Can you work these out from the model? Positions are in its coordinate system, mm. A direction names the side the tool comes from. Give positions to 0.01 mm unless a question says otherwise; leave off trailing zeros. Loops run counter-clockwise (first coordinate to the right, second up) from the corner with the lowest first, then second, coordinate; pieces in that order, holes last. Notation, with made-up numbers: (-37.75, 4) - (-7.75, 4) arc R30 ccw to (-7.75, 42) - close; hole circle Ø6 at (68, 88). An arc over 180 degrees is marked (long way). Answer as a JSON object with one key per item and string values. Group by question number.
Item 1: Suppose I cut it at B-B on x = 45.5. Write out the boundary of the cut face in (y, z), and give its area (3 significant figures).
Item 2: Suppose I cut it at A-A on y = 7.25. Write out the boundary of the cut face in (x, z), and give its area (3 significant figures).
Item 3: Thinking about a two-plate mould opening in X: for faces 1 (the flat face through (94.975, 10, 0)), 2 (the flat face through (78, 10, 25)), 3 (the flat face through (61.975, 10, 0)), which applies, pulls with the +X half, pulls with the -X half, needs draft (parallel to the pull), parting line crosses it, or undercut?
Item 4: Suppose I cut it at D-D on x = 8. Write out the boundary of the cut face in (y, z).
Item 5: Which directions (+Z, -Z, +X, -X, +Y, -Y) give clear straight access to the entire face, cutting with the end or side of a thin tool? Please do faces 4 (the flat face through (26.475, 10, 0)), 5 (the flat face through (78, 10, -25)), 6 (the flat face through (42, 10, 23)).
Item 6: Will these pins go through, and if not, where does the flat tip stop? pin 1 (5 mm diameter, centred on y = 9, z = -6.5, fed in from -X); pin 2 (3 mm diameter, centred on x = 73.5, y = 9, fed in from -Z); pin 3 (3 mm diameter, centred on y = 9, z = 9.5, fed in from +X).
Item 7: Suppose I cut it at C-C on z = 11.5. Write out the boundary of the cut face in (x, y).
Item 8: Please list where these lines run through material, in increasing order: L1, parallel to X at y = 8.75, z = 2.5; L2, parallel to Z at x = -33.5, y = 11.25; L3, parallel to Z at x = 43.5, y = 11.
from build123d import *

# Parameters (mm, degrees)
SKETCH1_W           = 165
SKETCH1_H           = 65
BOSS_EXTRUDE1_DEPTH = 5
FILLET1_R           = 5
SKETCH2_W           = 82
SKETCH2_H           = 55
SKETCH2_W_2         = 31
SKETCH2_H_2         = 46
SKETCH2_W_3         = 33
SKETCH2_H_3         = 50
BOSS_EXTRUDE2_DEPTH = 10
FILLET2_R           = 2
FILLET3_R           = 1


with BuildPart() as part:
    # Sketch1 → Boss-Extrude1 (new body)
    with BuildSketch(Plane(origin=(0, 0, 0), x_dir=(1, 0, 0), z_dir=(0, 1, 0))):
        with Locations((17.474934091, 0)):
            Rectangle(SKETCH1_W, SKETCH1_H)
    extrude(amount=BOSS_EXTRUDE1_DEPTH)

    # Fillet1
    fillet1_edges = [part.edges().sort_by_distance(p)[0] for p in [
        (-65.025065909, 2.5, -32.5),
        (99.974934091, 2.5, -32.5),
        (99.974934091, 2.5, 32.5),
        (-65.025065909, 2.5, 32.5),
    ]]
    fillet(fillet1_edges, radius=FILLET1_R)

    # Sketch2 → Boss-Extrude2 (add)
    with BuildSketch(Plane(origin=(0, 5, 0), x_dir=(1, 0, 0), z_dir=(0, 1, 0))):
        with Locations((-19.025065909, 0)):
            Rectangle(SKETCH2_W, SKETCH2_H)
        with Locations((41.974934091, 0)):
            Rectangle(SKETCH2_W_2, SKETCH2_H_2)
        with Locations((78.474934091, 0)):
            Rectangle(SKETCH2_W_3, SKETCH2_H_3)
    extrude(amount=BOSS_EXTRUDE2_DEPTH)

    # Fillet2
    fillet2_edges = [part.edges().sort_by_distance(p)[0] for p in [
        (26.474934091, 10, -23),
        (26.474934091, 10, 23),
        (57.474934091, 10, 23),
        (57.474934091, 10, -23),
    ]]
    fillet(fillet2_edges, radius=FILLET2_R)

    # Fillet3
    fillet3_edges = [part.edges().sort_by_distance(p)[0] for p in [
        (61.974934091, 10, -25),
        (61.974934091, 10, 25),
        (94.974934091, 10, 25),
        (94.974934091, 10, -25),
    ]]
    fillet(fillet3_edges, radius=FILLET3_R)


solid = part.part
Worked out:
{
 "1": {"outline": "(0, -32.5) - (5, -32.5) - (5, -23) - (15, -23) - (15, 23) - (5, 23) - (5, 32.5) - (0, 32.5) - close", "area": "785 mm2"},
 "2": {"outline": "(-60.03, -27.5) - (21.97, -27.5) - (21.97, 27.5) - (-60.03, 27.5) - close; (26.47, -21) arc R2 ccw to (28.47, -23) - (55.47, -23) arc R2 ccw to (57.47, -21) - (57.47, 21) arc R2 ccw to (55.47, 23) - (28.47, 23) arc R2 ccw to (26.47, 21) - close; (61.97, -24) arc R1 ccw to (62.97, -25) - (93.97, -25) arc R1 ccw to (94.97, -24) - (94.97, 24) arc R1 ccw to (93.97, 25) - (62.97, 25) arc R1 ccw to (61.97, 24) - close", "area": "7,580 mm2"},
 "3": {"face 1": "pulls with the +X half", "face 2": "needs draft", "face 3": "undercut"},
 "4": {"outline": "(0, -32.5) - (5, -32.5) - (5, -27.5) - (15, -27.5) - (15, 27.5) - (5, 27.5) - (5, 32.5) - (0, 32.5) - close"},
 "5": {"face 4": "+Z, -Z, +Y", "face 5": "-Z, +X, +Y", "face 6": "+Z, +Y"},
 "6": {"pin 1": "stops at x = -60.03", "pin 2": "stops at z = -25", "pin 3": "stops at x = 94.97"},
 "7": {"outline": "(-65.03, 0) - (99.97, 0) - (99.97, 5) - (94.97, 5) - (94.97, 15) - (61.97, 15) - (61.97, 5) - (57.47, 5) - (57.47, 15) - (26.47, 15) - (26.47, 5) - (21.97, 5) - (21.97, 15) - (-60.03, 15) - (-60.03, 5) - (-65.03, 5) - close"},
 "8": {"L1": "x = -60.03 to 21.97, 26.47 to 57.47, 61.97 to 94.97", "L2": "z = -27.5 to 27.5", "L3": "z = -23 to 23"}
}
